The listing builds one solid part. Answer for the finished solid, in the listing's coordinates (mm). Round coordinates to 2 decimals unless told otherwise and drop trailing zeros. Loops run counter-clockwise (first coordinate to the right, second up) from the corner with the lowest first, then second, coordinate; pieces in that order, holes last. Notation, with made-up numbers: (20, 8.5) - (62, 8.5) arc R5 ccw to (62, 17.5) - close; hole circle Ø8 at (-19.5, 38.25). An arc over 180 degrees is marked (long way). One line per item, written item: value.
```python
from build123d import *

# Parameters (mm, degrees)
F0_R     = 3.25
F1_DEPTH = 5


with BuildPart() as f1:
    # F0 (on Top) → F1 (new body)
    with BuildSketch(Plane.XY):
        Polygon((-43.508064, 47.219317), (-63.508064, 47.219317), (-63.508064, 40.219317), (-60.508064, 40.219317), (-60.508064, 30.219317), (-63.508064, 30.219317), (-63.508064, 23.219317), (-60.508064, 23.219317), (-60.508064, 13.219317), (-63.508064, 13.219317), (-63.508064, 6.219317), (-43.508064, 6.219317), (-43.508064, 3.219317), (-33.508064, 3.219317), (-33.508064, 6.219317), (-24.508064, 6.219317), (-24.508064, 12.219317), (-25.508064, 12.219317), (-25.508064, 14.219317), (-24.508064, 14.219317), (-24.508064, 18.219317), (-22.508064, 18.219317), (-22.508064, 14.219317), (-21.508064, 14.219317), (-21.508064, 12.219317), (-22.508064, 12.219317), (-22.508064, 6.219317), (-13.508064, 6.219317), (-13.508064, 3.219317), (-3.508064, 3.219317), (-3.508064, 6.219317), (5.491936, 6.219317), (5.491936, 12.219317), (4.491936, 12.219317), (4.491936, 14.219317), (5.491936, 14.219317), (5.491936, 18.219317), (7.491936, 18.219317), (7.491936, 14.219317), (8.491936, 14.219317), (8.491936, 12.219317), (7.491936, 12.219317), (7.491936, 6.219317), (16.491936, 6.219317), (16.491936, 3.219317), (26.491936, 3.219317), (26.491936, 6.219317), (46.491936, 6.219317), (46.491936, 13.219317), (43.491936, 13.219317), (43.491936, 23.219317), (46.491936, 23.219317), (46.491936, 30.219317), (43.491936, 30.219317), (43.491936, 40.219317), (46.491936, 40.219317), (46.491936, 47.219317), (26.491936, 47.219317), (26.491936, 50.219317), (16.491936, 50.219317), (16.491936, 47.219317), (7.491936, 47.219317), (7.491936, 41.219317), (8.491936, 41.219317), (8.491936, 39.219317), (7.491936, 39.219317), (7.491936, 35.219317), (5.491936, 35.219317), (5.491936, 39.219317), (4.491936, 39.219317), (4.491936, 41.219317), (5.491936, 41.219317), (5.491936, 47.219317), (-3.508064, 47.219317), (-3.508064, 50.219317), (-13.508064, 50.219317), (-13.508064, 47.219317), (-22.508064, 47.219317), (-22.508064, 41.219317), (-21.508064, 41.219317), (-21.508064, 39.219317), (-22.508064, 39.219317), (-22.508064, 35.219317), (-24.508064, 35.219317), (-24.508064, 39.219317), (-25.508064, 39.219317), (-25.508064, 41.219317), (-24.508064, 41.219317), (-24.508064, 47.219317), (-33.508064, 47.219317), (-33.508064, 50.219317), (-43.508064, 50.219317), align=None)
        with Locations((26.491936, 26.719317)):
            Circle(F0_R, mode=Mode.SUBTRACT)
    extrude(amount=F1_DEPTH)


solid = f1.part
```
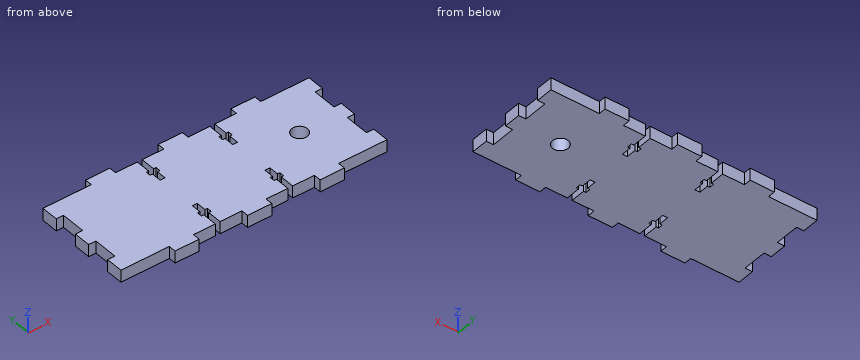
1) A cutting plane is placed at A-A on y = 43. Give the vertices of the cut face in (x, z).
Final values:
outline: (-63.51, 0) - (-24.51, 0) - (-24.51, 5) - (-63.51, 5) - close; (-22.51, 0) - (5.49, 0) - (5.49, 5) - (-22.51, 5) - close; (7.49, 0) - (46.49, 0) - (46.49, 5) - (7.49, 5) - close
2) A cutting plane is placed at B-B on y = 29. Give the vertices of the cut face in (x, z).
Final values:
outline: (-63.51, 0) - (24.18, 0) - (24.18, 5) - (-63.51, 5) - close; (28.81, 0) - (46.49, 0) - (46.49, 5) - (28.81, 5) - close
3) A cutting plane is placed at D-D on y = 15.5. Give the vertices of the cut face in (x, z), and give its area (3 significant figures).
Final values:
outline: (-60.51, 0) - (-24.51, 0) - (-24.51, 5) - (-60.51, 5) - close; (-22.51, 0) - (5.49, 0) - (5.49, 5) - (-22.51, 5) - close; (7.49, 0) - (43.49, 0) - (43.49, 5) - (7.49, 5) - close
area: 500 mm2
4) Each of these flat-tipped pins is pushed along its axis until it touches: pin 1 Ø0.5 at (x, z) = (-25, 2) entering from +Y; pin 2 Ø1.5 at (x, z) = (12, 1.5) entering from -Y; pin 3 Ø0.9 at (y, z) = (4.5, 3) entering from -X. Where does it stop, or does it pass through?
Final values:
pin 1: y = 47.22
pin 2: y = 6.22
pin 3: x = -43.51
5) A cutting plane is placed at C-C on x = 34.5. Give the vertices of the cut face in (y, z), and give its area (3 significant figures).
Final values:
outline: (6.22, 0) - (47.22, 0) - (47.22, 5) - (6.22, 5) - close
area: 205 mm2
6) Consider L1, parallel to X at y = 42.5, z = 3.5; L2, parallel to X at y = 17.5, z = 4.65; L3, parallel to Y at x = 15.5, z = 0.4. Determine where each line is inside the solid, lowest interval first.
Final values:
L1: -63.51 to -24.51, -22.51 to 5.49, 7.49 to 46.49
L2: -60.51 to -24.51, -22.51 to 5.49, 7.49 to 43.49
L3: 6.22 to 47.22
